Here's the drawing with two shaded views (mm, measured from the low corner). I have some questions. A direction names the side the tool comes from. Give positions to 0.01 mm unless a question says otherwise; leave off trailing zeros. Write each loop counter-clockwise with the first axis right and the second up, starting at its lowest first coordinate (ties: lowest second). Pieces come first, ordered by that corner, then holes. Notation, with made-up numbers: (71, 43.25) -> (128, 43.25) arc R27 ccw to (128, 63.25) -> close; hole circle Ø3 at (67, -4). An arc over 180 degrees is marked (long way). One line per item, written item: value.
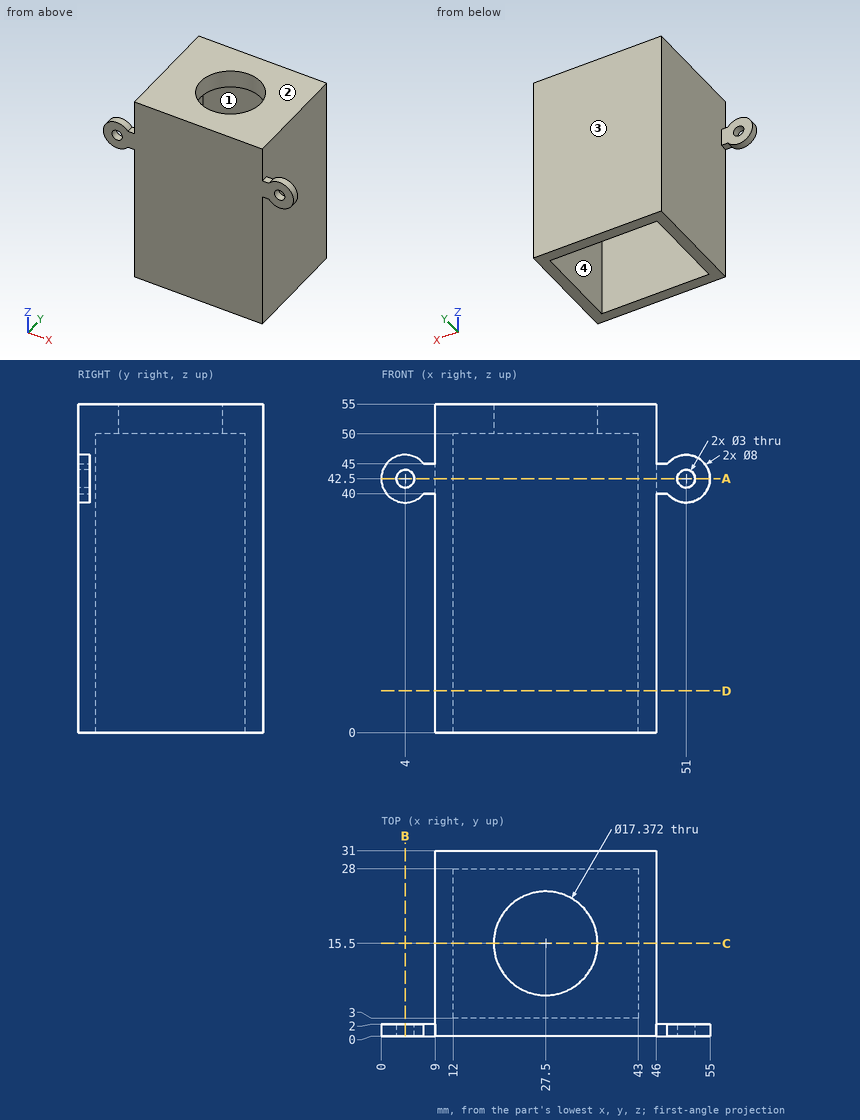
1) If we section it at D-D (z = 7): Write out the boundary of the cut face in (x, y).
Answer list:
outline: (9, 0) -> (46, 0) -> (46, 31) -> (9, 31) -> close; hole (12, 3) -> (43, 3) -> (43, 28) -> (12, 28) -> close
2) I need wall thicknesses on L1, parallel to X at y = 0.55, z = 42.5; L2, parallel to Y at x = 28, z = 32; L3, parallel to X at y = 15, z = 51. Which ranges of each line are inside material? Lowest first, please.
Answer list:
L1: x = 0 to 2.5, 5.5 to 49.5, 52.5 to 55
L2: y = 0 to 3, 28 to 31
L3: x = 9 to 18.83, 36.17 to 46
3) If we section it at A-A (z = 42.5): Write out the boundary of the cut face in (x, y), and give its area (3 significant figures).
Answer list:
outline: (0, 0) -> (2.5, 0) -> (2.5, 2) -> (0, 2) -> close; (5.5, 0) -> (49.5, 0) -> (49.5, 2) -> (46, 2) -> (46, 31) -> (9, 31) -> (9, 2) -> (5.5, 2) -> close; (52.5, 0) -> (55, 0) -> (55, 2) -> (52.5, 2) -> close; hole (12, 3) -> (43, 3) -> (43, 28) -> (12, 28) -> close
area: 396 mm^2
4) For the marked faces 1 and 2, which set-ups out of +Z, -Z, +X, -X, +Y, -Y let a thin tool reach every point of the face, with its end or its side?
Answer list:
face 1: -Z
face 2: +Z, +X, -X, +Y, -Y
5) We'd pull the mould along X, two halves only. Please class the marked faces 3 and 4: released by +X, released by -X, zero draft, split by the parting line, or undercut.
Answer list:
face 3: zero draft
face 4: undercut
6) If we section it at B-B (x = 4): Write out the boundary of the cut face in (y, z).
Answer list:
outline: (0, 38.5) -> (2, 38.5) -> (2, 41) -> (0, 41) -> close; (0, 44) -> (2, 44) -> (2, 46.5) -> (0, 46.5) -> close
7) Will these pins go through, and if not, where does the flat tip stop? pin 1 (2.5 mm diameter, centred on x = 3, z = 43.5, fed in from +Y); pin 2 (1 mm diameter, centred on y = 14, z = 40.5, fed in from -X); pin 3 (8 mm diameter, centred on y = 19, z = 6.5, fed in from +X); pin 4 (1.5 mm diameter, centred on x = 7, y = 11, fed in from -Z).
Answer list:
pin 1: stops at y = 2
pin 2: stops at x = 9
pin 3: stops at x = 46
pin 4: passes through
8) If we section it at C-C (y = 15.5): Write out the boundary of the cut face in (x, z).
Answer list:
outline: (9, 0) -> (12, 0) -> (12, 50) -> (18.81, 50) -> (18.81, 55) -> (9, 55) -> close; (36.19, 50) -> (43, 50) -> (43, 0) -> (46, 0) -> (46, 55) -> (36.19, 55) -> close
